```python
from build123d import *

# Parameters (mm, degrees)
SKETCH_1_W          = 260
SKETCH_1_H          = 205
SKETCH_1_W_2        = 252
SKETCH_1_H_2        = 197
EXTRUDE_1_DEPTH     = 140
SKETCH_2_W          = 260
SKETCH_2_H          = 205
EXTRUDE_1_2_DEPTH   = 5
SKETCH_3_R          = 10
CUT_EXTRUDE_1_DEPTH = 5
CHAMFER_1_SIZE      = 80
CHAMFER_1_SIZE2     = 29.117618741
CHAMFER_2_SIZE      = 110
CHAMFER_2_SIZE2     = 40.036725769
FILLET_1_R          = 15


with BuildPart() as part:
    # 草图1 → Extrude 1 (new body)
    with BuildSketch(Plane.XY):
        Rectangle(SKETCH_1_W, SKETCH_1_H)
        Rectangle(SKETCH_1_W_2, SKETCH_1_H_2, mode=Mode.SUBTRACT)
    extrude(amount=EXTRUDE_1_DEPTH)

    # 草图2 → Extrude 1 2 (add)
    with BuildSketch(Plane(origin=(0, 0, 0), x_dir=(-1, 0, 0), z_dir=(0, 0, -1))):
        Rectangle(SKETCH_2_W, SKETCH_2_H)
    extrude(amount=-EXTRUDE_1_2_DEPTH)

    # 草图3 → 切除-拉伸1 (cut)
    with BuildSketch(Plane(origin=(0, 0, 0), x_dir=(-1, 0, 0), z_dir=(0, 0, -1))):
        Circle(SKETCH_3_R)
    extrude(amount=-CUT_EXTRUDE_1_DEPTH, mode=Mode.SUBTRACT)

    # 倒角1
    chamfer_1_edges = [part.edges().sort_by_distance(p)[0] for p in [
        (0, -98.5, 5),
        (0, 98.5, 5),
    ]]
    chamfer_1_side = [part.faces().sort_by_distance(p)[0] for p in [
        (122.801359664, 0, 5),
    ]]
    chamfer(chamfer_1_edges, length=CHAMFER_1_SIZE, length2=CHAMFER_1_SIZE2, reference=chamfer_1_side[0])

    # 倒角2
    chamfer_2_edges = [part.edges().sort_by_distance(p)[0] for p in [
        (-126, 0, 5),
        (126, 0, 5),
    ]]
    chamfer_2_side = [part.faces().sort_by_distance(p)[0] for p in [
        (123.452982136, 0, 5),
    ]]
    chamfer(chamfer_2_edges, length=CHAMFER_2_SIZE, length2=CHAMFER_2_SIZE2, reference=chamfer_2_side[0])

    # 圆角1
    fillet_1_edges = [part.edges().sort_by_distance(p)[0] for p in [
        (56, 58.5, 19.558809371),
        (-56, 58.5, 19.558809371),
        (56, -58.5, 19.558809371),
        (-56, -58.5, 19.558809371),
    ]]
    fillet(fillet_1_edges, radius=FILLET_1_R)


solid = part.part
```
Work out the finished part from the listing and answer in its coordinate system (mm). A direction names the side the tool comes from. Give positions to 0.01 mm unless a question says otherwise; leave off trailing zeros. Order: outer loops, then holes, each group sorted by start corner. A loop starts at its lowest first (then second) coordinate and runs counter-clockwise, first axis right, second up.
1. Each of these flat-tipped pins is pushed along its axis until it touches: P1, Ø6, axis at x = -99.5, y = -62.5, coming from the +Z side; P2, Ø16, axis at x = 0, y = 0, coming from the -Z side; P3, Ø2, axis at x = -47, y = -71.5, coming from the +Z side. Where does it stop, or does it pass through?
Result sheet:
P1: stops at z = 36.48
P2: passes through
P3: stops at z = 24.65
2. For faces 1 (the cylindrical face through (56.71, -59.14, 20.28)), 2 (the cylindrical face through (2.17, -9.76, 2.46)), determine the directions among +Z, -Z, +X, -X, +Y, -Y from which every point of the face is accessible in a straight line to the end or side of a thin tool.
Result sheet:
face 1: +Z
face 2: +Z, -Z
3. Section B-B, the plane x = 0 is taken. Determine the outline of the cut face in (y, z), and give its area (3 significant figures).
Result sheet:
outline: (-102.5, 0) - (-10, 0) - (-10, 5) - (-18.5, 5) - (-98.5, 34.12) - (-98.5, 140) - (-102.5, 140) - close; (10, 0) - (102.5, 0) - (102.5, 140) - (98.5, 140) - (98.5, 34.12) - (18.5, 5) - (10, 5) - close
area: 4,330 mm2
4. Straight lines are drawn through the part: L1, parallel to Y at x = 56, z = 80.5; L2, parallel to X at y = 78.5, z = 113.5; L3, parallel to Y at x = 0, z = 2.5. For each, find the intervals that lie inside material, in ascending order.
Result sheet:
L1: y = -102.5 to -98.5, 98.5 to 102.5
L2: x = -130 to -126, 126 to 130
L3: y = -102.5 to -10, 10 to 102.5
5. Section A-A, the plane y = 0 is taken. Determine the outline of the cut face in (x, z), and give its area (3 significant figures).
Result sheet:
outline: (-130, 0) - (-10, 0) - (-10, 5) - (-16, 5) - (-126, 45.04) - (-126, 140) - (-130, 140) - close; (10, 0) - (130, 0) - (130, 140) - (126, 140) - (126, 45.04) - (16, 5) - (10, 5) - close
area: 6,680 mm2
6. Section C-C, the plane z = 123 is taken. Determine the outline of the cut face in (x, y).
Result sheet:
outline: (-130, -102.5) - (130, -102.5) - (130, 102.5) - (-130, 102.5) - close; hole (-126, -98.5) - (126, -98.5) - (126, 98.5) - (-126, 98.5) - close
